from build123d import *

# Parameters (mm, degrees)
F1_DEPTH = 10
F2_R     = 2
F3_DEPTH = 15.326
F4_R     = 5
F5_R     = 1.49999


# Not quite as in the source:
# - a fillet or chamfer is up to 0.001 mm smaller than in the source, because OpenCascade refuses the exact size


with BuildPart() as f1:
    # F0 (on Top) → F1 (new body)
    with BuildSketch(Plane.XY):
        with BuildLine():
            Line((-15.0284937702, 3), (-27.325, 3))
            Line((-27.325, 3), (-27.325, 0))
            Line((-27.325, 0), (-12.825, 0))
            ThreePointArc((-12.825, 0), (0, 12.825), (12.825, 0))
            Line((12.825, 0), (27.325, 0))
            Line((27.325, 0), (27.325, 3))
            Line((27.325, 3), (15.0284937702, 3))
            ThreePointArc((15.0284937702, 3), (0, 15.325), (-15.0284937702, 3))
        make_face()
    extrude(amount=F1_DEPTH)

    # F2 (on face) → F3 (cut, through all)
    with BuildSketch(Plane.XZ):
        with Locations((-22.325, 5)):
            Circle(F2_R)
        with Locations((22.325, 5)):
            Circle(F2_R)
    extrude(amount=-F3_DEPTH, mode=Mode.SUBTRACT)

    # F4
    f4_edges = [f1.edges().sort_by_distance(p)[0] for p in [
        (-15.028494, 3, 5),
        (15.028494, 3, 5),
    ]]
    fillet(f4_edges, radius=F4_R)

    # F5 (radius 1.5 in the source; OpenCascade refuses exactly that, so slightly less here)
    f5_edges = [f1.edges().sort_by_distance(p)[0] for p in [
        (-27.325, 0, 5),
        (-27.325, 3, 5),
        (27.325, 0, 5),
        (27.325, 3, 5),
    ]]
    fillet(f5_edges, radius=F5_R)


solid = f1.part
CAD build for the part. Positions are in the model's coordinates, mm. A direction names the side the tool comes from. Round coordinates to 2 decimals unless told otherwise and drop trailing zeros. Loops run counter-clockwise (first coordinate to the right, second up) from the corner with the lowest first, then second, coordinate; pieces in that order, holes last. Notation, with made-up numbers: (5, 47) - (52, 47) arc R14 ccw to (52, 61) - close; hole circle Ø10 at (79.5, -7). An arc over 180 degrees is marked (long way). Put each result on its own line as item: value.
1. Wall check: line 1 (Y direction, x = -23.5, z = 6.75); line 2 (X direction, y = 9, z = 1.25); line 3 (X direction, y = 5.5, z = 4). Give the ranges that are in metal, low to high.
Geometry check:
line 1: 0 to 3
line 2: -12.4 to -9.14, 9.14 to 12.4
line 3: -14.35 to -11.59, 11.59 to 14.35
2. Two-plate mould, pull along Z, no slides. Class faces 4 (the flat face through (-2, 13, 10)), 5 (the cylindrical face through (-0.28, 12.82, 4.93)), 6 (the cylindrical face through (24.233, 1.479, 5.601)), 7 (the flat face through (-2, 13, 0)): released by +Z, released by -Z, zero draft, split by the parting line, or undercut.
Geometry check:
face 4: released by +Z
face 5: zero draft
face 6: undercut
face 7: released by -Z
3. Slice it at A-A on z = 5. Give the number of separate pieces and of enclosed holes in the cut face, and give its area (3 significant figures).
Geometry check:
separate pieces: 3
enclosed holes: 0
area: 162 mm²
4. 3-axis set-ups, long thin cutter, end or side, ignore diameter. For faces 1 (the flat face through (-22.2, 3, 2.7)), 2 (the cylindrical face through (0.25, 15.323, 4.93)), 3 (the flat face through (22.3, 3, 2.7)): which of +Z, -Z, +X, -X, +Y, -Y reach the whole face in a straight line?
Geometry check:
face 1: +Z, -Z, -X, +Y
face 2: +Z, -Z, +Y
face 3: +Z, -Z, +X, +Y
5. Slice it at B-B on y = 11.5. List the corners of the cut face in (x, z), and give its area (3 significant figures).
Geometry check:
outline: (-10.13, 0) - (-5.68, 0) - (-5.68, 10) - (-10.13, 10) - close; (5.68, 0) - (10.13, 0) - (10.13, 10) - (5.68, 10) - close
area: 89.0 mm²
6. Pin check, flat tips, straight feed: P1, Ø5.5, axis at x = -23.5, z = 7.5, coming from the +Y side; P2, Ø4, axis at x = -15.5, y = 1.5, coming from the -Z side. Stop position of each tip, or through.
Geometry check:
P1: y = 3
P2: z = 0
7. Slice it at C-C on x = -22.5. List the corners of the cut face in (y, z).
Geometry check:
outline: (0, 0) - (3, 0) - (3, 3.01) - (0, 3.01) - close; (0, 6.99) - (3, 6.99) - (3, 10) - (0, 10) - close
